The listing builds one solid part. Answer for the finished solid, in the listing's coordinates (mm). Face numbers are marked on the shaded views. A direction names the side the tool comes from. Coordinates: 2 decimals unless noted, no trailing zeros. Write each loop counter-clockwise with the first axis right and the second up, starting at its lowest first coordinate (ties: lowest second). Pieces come first, ordered by that corner, then holes.
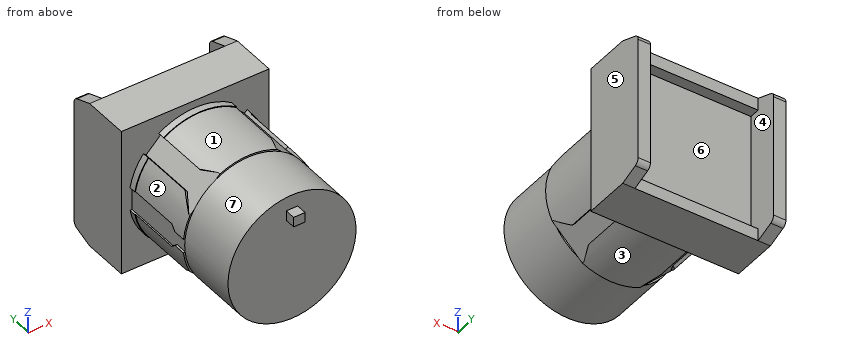
Autodesk Inventor part; units mm, degrees
ref_plane "body_to_cap_XY" through (0, 4.318, 0) normal (0, 1, 0) x (1, 0, 0)
ref_plane "body_to_cap_YZ" through (0, 4.318, 0) normal (1, 0, 0) x (0, 0, -1)
ref_plane "body_to_cap_ZX" through (0, 4.318, 0) normal (0, 0, -1) x (0, 1, 0)
sketch "Sketch_1" plane through (0, 0, 0) normal (0, 0, 1) x (1, 0, 0)
  line L0 (0, 0) -> (0, -9.398)
  line L1 (0, -9.398) -> (-8, -9.398)
  line L2 (-8, -9.398) -> (-8, -0.8382)
  line L3 (-8, -0.8382) -> (-8.0808, -0.8382)
  line L4 (-8.0808, -0.8382) -> (-8.0808, 0)
  line L5 (-8.0808, 0) -> (0, 0)
  line L6 (0, 0) -> (0, -9.398)
revolve "Revolution1" add sketch "Sketch_1" angle 360 about axis through (0, 0, 0) along (0, 1, 0)
thread "Thread1"
sketch "Sketch_15" plane through (0, 0, 0) normal (0, 0, 1) x (1, 0, 0)
  line L0 (0, -9.398) -> (0, -16.9926)
  line L1 (0, -16.9926) -> (-7.8049, -16.9926)
  line L2 (-7.8049, -16.9926) -> (-7.8049, -9.398)
  line L3 (-7.8049, -9.398) -> (0, -9.398)
  line L4 (0, -9.398) -> (0, -16.9926)
revolve "Revolution2" add sketch "Sketch_15" angle 360 about axis through (0, -9.398, 0) along (0, 1, 0)
sketch "Sketch_7" plane through (-5.714, 0, 5.714) normal (0.7071, 0, -0.7071) x (-0.7071, 0, -0.7071)
  line L0 (-2.7242, -9.398) -> (2.7242, -9.398)
  line L1 (2.7242, -9.398) -> (0.9081, -7.2337)
  line L2 (0.9081, -7.2337) -> (0.9081, 0)
  line L3 (0.9081, 0) -> (-1.6345, 0)
  line L4 (-1.6345, 0) -> (-1.6345, -7.0612)
  line L5 (-1.6345, -7.0612) -> (-2.7242, -9.398)
extrude "Extrusion1" cut sketch "Sketch_7" along normal blind 0.508
sketch "Sketch_9" plane through (5.714, 0, 5.714) normal (0.7071, 0, 0.7071) x (0.7071, 0, -0.7071)
  line L0 (-2.7242, -9.398) -> (2.7242, -9.398)
  line L1 (2.7242, -9.398) -> (0.9081, -7.2337)
  line L2 (0.9081, -7.2337) -> (0.9081, 0)
  line L3 (0.9081, 0) -> (-1.6345, 0)
  line L4 (-1.6345, 0) -> (-1.6345, -7.0612)
  line L5 (-1.6345, -7.0612) -> (-2.7242, -9.398)
extrude "Extrusion2" cut sketch "Sketch_9" against normal blind 0.508
sketch "Sketch_8" plane through (5.714, 0, -5.714) normal (0.7071, 0, -0.7071) x (-0.7071, 0, -0.7071)
  line L0 (-2.7242, -9.398) -> (2.7242, -9.398)
  line L1 (2.7242, -9.398) -> (1.6345, -7.0612)
  line L2 (1.6345, -7.0612) -> (1.6345, 0)
  line L3 (1.6345, 0) -> (-0.9081, 0)
  line L4 (-0.9081, 0) -> (-0.9081, -7.2337)
  line L5 (-0.9081, -7.2337) -> (-2.7242, -9.398)
extrude "Extrusion3" cut sketch "Sketch_8" against normal blind 0.508
sketch "Sketch_10" plane through (-5.714, 0, -5.714) normal (0.7071, 0, 0.7071) x (0.7071, 0, -0.7071)
  line L0 (-2.7242, -9.398) -> (2.7242, -9.398)
  line L1 (2.7242, -9.398) -> (1.6345, -7.0612)
  line L2 (1.6345, -7.0612) -> (1.6345, 0)
  line L3 (1.6345, 0) -> (-0.9081, 0)
  line L4 (-0.9081, 0) -> (-0.9081, -7.2337)
  line L5 (-0.9081, -7.2337) -> (-2.7242, -9.398)
extrude "Extrusion4" cut sketch "Sketch_10" along normal blind 0.508
sketch "Sketch_14" plane through (-8.2051, 0, 0) normal (1, 0, 0) x (0, 0, -1)
  line L0 (-1.4346, -7.2187) -> (-0.8534, -7.9113)
  line L1 (-0.8534, -7.9113) -> (-0.8534, -9.398)
  line L2 (-0.8534, -9.398) -> (0.8534, -9.398)
  line L3 (0.8534, -9.398) -> (0.8534, -7.9113)
  line L4 (0.8534, -7.9113) -> (1.4346, -7.2187)
  line L5 (1.4346, -7.2187) -> (1.4346, 0)
  line L6 (1.4346, 0) -> (-1.4346, 0)
  line L7 (-1.4346, 0) -> (-1.4346, -7.2187)
extrude "Extrusion5" cut sketch "Sketch_14" along normal blind 0.508
sketch "Sketch_20" plane through (0, 0, 0) normal (1, 0, 0) x (0, 1, 0)
  line L0 (0, 9.0043) -> (0, -9.0043)
  line L1 (0, -9.0043) -> (5.588, -9.0043)
  line L2 (5.588, -9.0043) -> (7.8044, -8.1976)
  arc A0 (7.8044, -8.1976) -> (8.3058, -7.4815) centre (7.5438, -7.4815) ccw
  line L3 (8.3058, -7.4815) -> (8.3058, 7.4815)
  arc A1 (8.3058, 7.4815) -> (7.8044, 8.1976) centre (7.5438, 7.4815) ccw
  line L4 (7.8044, 8.1976) -> (5.588, 9.0043)
  line L5 (5.588, 9.0043) -> (0, 9.0043)
extrude "Extrusion6" add sketch "Sketch_20" along normal mid plane 18.0086
sketch "Sketch_19" plane through (0, 0, 0) normal (0, 0, 1) x (1, 0, 0)
  line L0 (-7.5057, 5.588) -> (7.5057, 5.588)
  line L1 (7.5057, 5.588) -> (7.5057, 9.5758)
  line L2 (7.5057, 9.5758) -> (-7.5057, 9.5758)
  line L3 (-7.5057, 9.5758) -> (-7.5057, 5.588)
extrude "Extrusion7" cut sketch "Sketch_19" along normal mid plane 30.0228
sketch "Sketch_18" plane through (0, 4.318, 0) normal (0, 1, 0) x (1, 0, 0)
  line L0 (-7.5057, 7.5057) -> (-7.5057, -7.5057)
  line L1 (-7.5057, -7.5057) -> (7.5057, -7.5057)
  line L2 (7.5057, -7.5057) -> (7.5057, 7.5057)
  line L3 (7.5057, 7.5057) -> (-7.5057, 7.5057)
extrude "Extrusion8" cut sketch "Sketch_18" along normal blind 8.3058
sketch "Sketch_2" plane through (0, -16.9926, 0) normal (0, 1, 0) x (1, 0, 0)
  line L0 (-0.7, -6.096) -> (0.7, -6.096)
  line L1 (0.7, -6.096) -> (0.7, -4.896)
  line L2 (0.7, -4.896) -> (-0.7, -4.896)
  line L3 (-0.7, -4.896) -> (-0.7, -6.096)
extrude "Extrusion9" add sketch "Sketch_2" along normal mid plane 2.6
ref_plane "body_to_cap_XY" through (0, 4.318, 0) normal (0, 1, 0) x (1, 0, 0)
ref_plane "body_to_cap_YZ" through (0, 4.318, 0) normal (1, 0, 0) x (0, 0, -1)
ref_plane "body_to_cap_ZX" through (0, 4.318, 0) normal (0, 0, -1) x (0, 1, 0)
ref_plane "body_to_metal_XY" through (0, -8.7173, 0) normal (0, 1, 0) x (1, 0, 0)
ref_plane "body_to_metal_YZ" through (0, -8.7173, 0) normal (1, 0, 0) x (0, 0, -1)
ref_plane "body_to_metal_ZX" through (0, -8.7173, 0) normal (0, 0, -1) x (0, 1, 0)
ref_plane "body_to_nut_XY" through (0, 0, 0) normal (0, 1, 0) x (1, 0, 0)
ref_plane "body_to_nut_YZ" through (0, 0, 0) normal (1, 0, 0) x (0, 0, -1)
ref_plane "body_to_nut_ZX" through (0, 0, 0) normal (0, 0, -1) x (0, 1, 0)
properties part number "YB16SKW01-BBni_body"
Q1. Given pin 1 (8 mm diameter, centred on y = -0.5, z = 1.5, fed in from +X); pin 2 (1 mm diameter, centred on y = -7.5, z = -3, fed in from -X); pin 3 (3 mm diameter, centred on x = 5, z = 5.5, fed in from +Y); pin 4 (1.5 mm diameter, centred on x = 7, y = -15.5, fed in from +Z), each flat-ended and moving along its own axis, determine where each tip first touches the part or whether it passes through.
Answers below:
pin 1: stops at x = 9
pin 2: stops at x = -7.6
pin 3: stops at y = 4.32
pin 4: stops at z = 4.67
Q2. Which of the six approach directions +Z, -Z, +X, -X, +Y, -Y give full straight-line access (tool end or side, diameter ignored) to the marked faces 1, 2 and 3?
Answers below:
face 1: +Z, -Y
face 2: +Z, -X, -Y
face 3: -Z, -Y
Q3. The part is cut by section A-A, the plane z = 0. Write down the section's boundary in (x, y).
Answers below:
outline: (-9, 0) - (-7.7, 0) - (-7.7, -9.4) - (-7.8, -9.4) - (-7.8, -16.99) - (7.8, -16.99) - (7.8, -9.4) - (8, -9.4) - (8, -0.84) - (8.08, -0.84) - (8.08, 0) - (9, 0) - (9, 8.31) - (7.51, 8.31) - (7.51, 4.32) - (-7.51, 4.32) - (-7.51, 8.31) - (-9, 8.31) - close
Q4. Find the intervals of material crossed by probe 1 along X at (y, z) = (6, -4.25); probe 2 along Y at (x, z) = (-2.5, 3), in increasing order.
Answers below:
probe 1: x = -9 to -7.51, 7.51 to 9
probe 2: y = -16.99 to 4.32
Q5. The part is cut by section C-C, the plane y = -4.5. Write down the section's boundary in (x, z), then the cut area to 3 significant figures.
Answers below:
outline: (-7.87, -1.43) arc R8 ccw to (-6.26, -4.98) - (-6, -4.71) - (-4.2, -6.51) - (-4.38, -6.69) arc R8 ccw to (4.38, -6.69) - (4.2, -6.51) - (6, -4.71) - (6.26, -4.98) arc R8 ccw to (6.26, 4.98) - (6, 4.71) - (4.2, 6.51) - (4.38, 6.69) arc R8 ccw to (-4.38, 6.69) - (-4.2, 6.51) - (-6, 4.71) - (-6.26, 4.98) arc R8 ccw to (-7.87, 1.43) - (-7.7, 1.43) - (-7.7, -1.43) - close
area: 196 mm2
Q6. The part is cut by section D-D, the plane y = -16. Write down the section's boundary in (x, z).
Answers below:
outline: circle Ø15.61 at (0, 0)
Q7. The part is cut by section B-B, the plane x = -1.5. Write down the section's boundary in (y, z).
Answers below:
outline: (-16.99, -7.66) - (-9.4, -7.66) - (-9.4, -7.86) - (-0.84, -7.86) - (-0.84, -7.94) - (0, -7.94) - (0, -9) - (5.59, -9) - (5.59, -7.51) - (4.32, -7.51) - (4.32, 7.51) - (5.59, 7.51) - (5.59, 9) - (0, 9) - (0, 7.94) - (-0.84, 7.94) - (-0.84, 7.86) - (-9.4, 7.86) - (-9.4, 7.66) - (-16.99, 7.66) - close
Q8. Determine the mould class of the marked faces 4, 5, 6 and 7 for opening direction X: released by +X, released by -X, zero draft, split by the parting line, or undercut.
Answers below:
face 4: undercut
face 5: released by +X
face 6: undercut
face 7: split by the parting line
